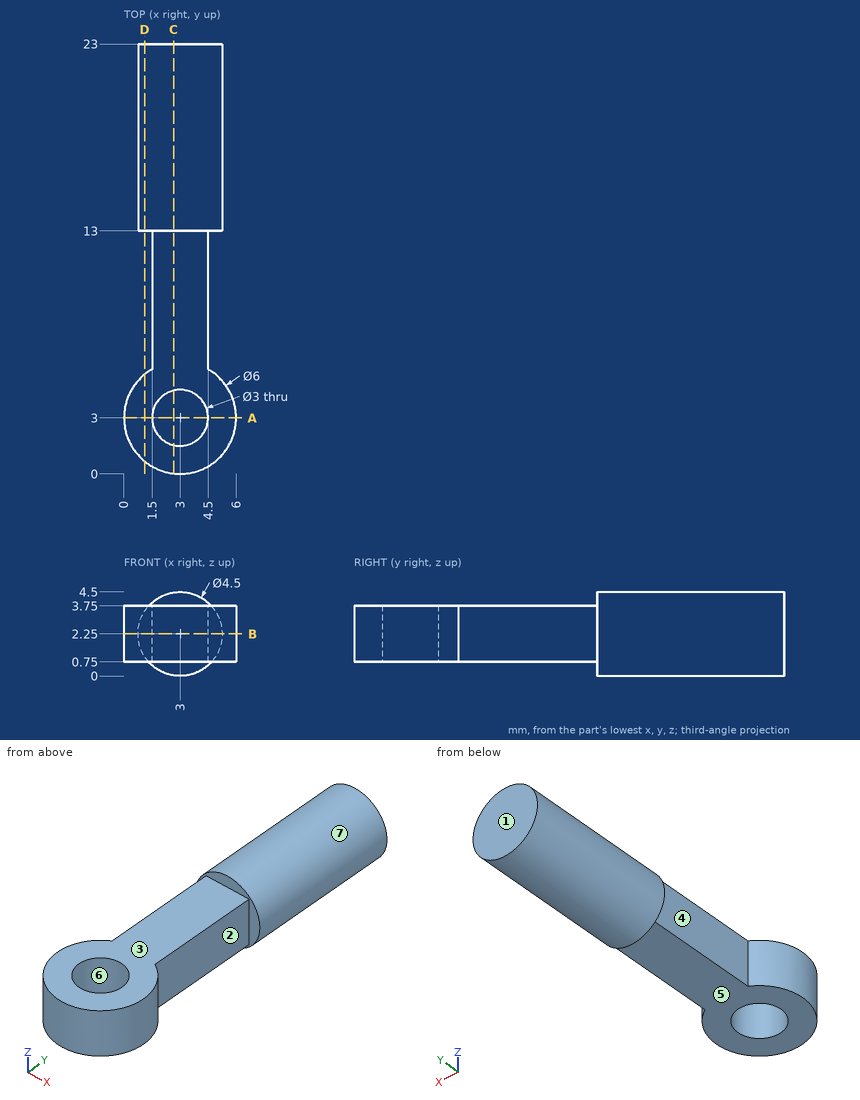
Verification items for this drawing (mm, ordinates from the low corner). A direction names the side the tool comes from. Coordinates: 2 decimals unless noted, no trailing zeros. Order: outer loops, then holes, each group sorted by start corner. A loop starts at its lowest first (then second) coordinate and runs counter-clockwise, first axis right, second up. Notation, with made-up numbers: M 25,-37 L 36,-37 A20 ccw 36,-18 Z; hole C 57.25,10 d9. An arc over 180 degrees is marked long. Answer as a JSON object with one key per item and string values.
Q1. Tool access check on the marked faces 5, 6 and 7. Record the directions out of +Z, -Z, +X, -X, +Y, -Y that give a thin tool (end or side, any length) a straight path to the whole face; none if there is none.
Results are:
{"face 5": "-Z, +X, -X, -Y", "face 6": "+Z, -Z", "face 7": "+Y"}
Q2. Cross-section at D-D on x = 1.1. Record the cut outline in (y, z), and give its area (3 significant figures).
Results are:
{"outline": "M 0.68,0.75 L 5.32,0.75 L 5.32,3.75 L 0.68,3.75 Z; M 13,1.04 L 23,1.04 L 23,3.46 L 13,3.46 Z", "area": "38.0 mm²"}
Q3. Depth check by flat-ended pin: pin 1 Ø1.8 at (x, y) = (4.5, 3.5) entering from +Z; pin 2 Ø2 at (x, y) = (5, 13) entering from -Z; pin 3 Ø1.5 at (y, z) = (8.5, 2) entering from -X. Enter the tip coordinate at first touch or a pass-through.
Results are:
{"pin 1": "stops at z = 3.75", "pin 2": "stops at z = 0.23", "pin 3": "stops at x = 1.5"}
Q4. Cross-section at C-C on x = 2.65. Record the cut outline in (y, z), and give its area (3 significant figures).
Results are:
{"outline": "M 0.02,0.75 L 1.54,0.75 L 1.54,3.75 L 0.02,3.75 Z; M 4.46,0.75 L 13,0.75 L 13,0.03 L 23,0.03 L 23,4.47 L 13,4.47 L 13,3.75 L 4.46,3.75 Z", "area": "74.6 mm²"}
Q5. Release check for a two-part mould opening along Y. For the marked faces 1, 2, 3 and 4 record: released by +Y, released by -Y, zero draft, split by the parting line, or undercut.
Results are:
{"face 1": "released by +Y", "face 2": "undercut", "face 3": "zero draft", "face 4": "undercut"}
Q6. Cross-section at B-B on z = 2.25. Record the cut outline in (x, y).
Results are:
{"outline": "M 0.75,13 L 1.5,13 L 1.5,5.6 A3 ccw long 4.5,5.6 L 4.5,13 L 5.25,13 L 5.25,23 L 0.75,23 Z; hole C 3,3 d3"}
Q7. Cross-section at A-A on y = 3. Record the cut outline in (x, z), and give its area (3 significant figures).
Results are:
{"outline": "M 0,0.75 L 1.5,0.75 L 1.5,3.75 L 0,3.75 Z; M 4.5,0.75 L 6,0.75 L 6,3.75 L 4.5,3.75 Z", "area": "9.00 mm²"}
Q8. Scan lines: line 1 (Y direction, x = 3, z = 2.6); line 2 (Z direction, x = 4.05, y = 12.5); line 3 (Y direction, x = 4.15, z = 2.5). Record each from-to range of solid material in increasing order.
Results are:
{"line 1": "y = 0 to 1.5, 4.5 to 23", "line 2": "z = 0.75 to 3.75", "line 3": "y = 0.23 to 2.04, 3.96 to 23"}
